from build123d import *

# Parameters (mm, degrees)
SKETCH1_R           = 2.1
SKETCH1_W           = 55.2
SKETCH1_H           = 5.05
BOSS_EXTRUDE1_DEPTH = 5
SKETCH2_W           = 55.4
SKETCH2_H           = 5.4
CUT_EXTRUDE1_DEPTH  = 10
SKETCH3_W           = 52.4
SKETCH3_H           = 5
CUT_EXTRUDE2_DEPTH  = 10
SKETCH4_W           = 40
SKETCH4_H           = 105
CUT_EXTRUDE3_DEPTH  = 10


with BuildPart() as part:
    # Sketch1 → Boss-Extrude1 (new body)
    with BuildSketch(Plane.XY):
        with BuildLine():
            Line((-192, 100.877501001), (-192, 60.122498999))
            ThreePointArc((-192, 60.122498999), (-193.5, 57), (-192, 53.877501001))
            Line((-192, 53.877501001), (-192, 13.122498999))
            ThreePointArc((-192, 13.122498999), (-193.5, 10), (-192, 6.877501001))
            Line((-192, 6.877501001), (-192, 0))
            Line((-192, 0), (-122, 0))
            Line((-122, 0), (-122, 5))
            Line((-122, 5), (-98.1, 5))
            Line((-98.1, 5), (-98.1, 11.8))
            Line((-98.1, 11.8), (-99.5, 11.8))
            Line((-99.5, 11.8), (-99.5, 15))
            Line((-99.5, 15), (-98.1, 15))
            Line((-98.1, 15), (-98.1, 22))
            Line((-98.1, 22), (-93.9, 22))
            Line((-93.9, 22), (-93.9, 15))
            Line((-93.9, 15), (-92.5, 15))
            Line((-92.5, 15), (-92.5, 11.8))
            Line((-92.5, 11.8), (-93.9, 11.8))
            Line((-93.9, 11.8), (-93.9, 5))
            Line((-93.9, 5), (-70, 5))
            Line((-70, 5), (-70, 0))
            Line((-70, 0), (0, 0))
            Line((0, 0), (0, 30.327501001))
            ThreePointArc((0, 30.327501001), (1.5, 33.45), (0, 36.572498999))
            Line((0, 36.572498999), (0, 77.327501001))
            ThreePointArc((0, 77.327501001), (1.5, 80.45), (0, 83.572498999))
            Line((0, 83.572498999), (0, 122.277501001))
            ThreePointArc((0, 122.277501001), (1.5, 125.4), (0, 128.522498999))
            Line((0, 128.522498999), (0, 160))
            Line((0, 160), (-32.9, 160))
            Line((-32.9, 160), (-32.9, 153.2))
            Line((-32.9, 153.2), (-31.5, 153.2))
            Line((-31.5, 153.2), (-31.5, 150))
            Line((-31.5, 150), (-32.9, 150))
            Line((-32.9, 150), (-32.9, 143))
            Line((-32.9, 143), (-37.1, 143))
            Line((-37.1, 143), (-37.1, 150))
            Line((-37.1, 150), (-38.5, 150))
            Line((-38.5, 150), (-38.5, 153.2))
            Line((-38.5, 153.2), (-37.1, 153.2))
            Line((-37.1, 153.2), (-37.1, 160))
            Line((-37.1, 160), (-154.9, 160))
            Line((-154.9, 160), (-154.9, 153.2))
            Line((-154.9, 153.2), (-153.5, 153.2))
            Line((-153.5, 153.2), (-153.5, 150))
            Line((-153.5, 150), (-154.9, 150))
            Line((-154.9, 150), (-154.9, 143))
            Line((-154.9, 143), (-159.1, 143))
            Line((-159.1, 143), (-159.1, 150))
            Line((-159.1, 150), (-160.5, 150))
            Line((-160.5, 150), (-160.5, 153.2))
            Line((-160.5, 153.2), (-159.1, 153.2))
            Line((-159.1, 153.2), (-159.1, 160))
            Line((-159.1, 160), (-192, 160))
            Line((-192, 160), (-192, 107.122498999))
            ThreePointArc((-192, 107.122498999), (-193.5, 104), (-192, 100.877501001))
        make_face()
        with Locations((-189.5, 104)):
            Circle(SKETCH1_R, mode=Mode.SUBTRACT)
        with Locations((-189.5, 57)):
            Circle(SKETCH1_R, mode=Mode.SUBTRACT)
        with Locations((-189.5, 10)):
            Circle(SKETCH1_R, mode=Mode.SUBTRACT)
        with Locations((-2.5, 125.4)):
            Circle(SKETCH1_R, mode=Mode.SUBTRACT)
        with Locations((-2.5, 80.45)):
            Circle(SKETCH1_R, mode=Mode.SUBTRACT)
        with Locations((-2.5, 33.45)):
            Circle(SKETCH1_R, mode=Mode.SUBTRACT)
        with Locations((-159.4, 127.475)):
            Rectangle(SKETCH1_W, SKETCH1_H, mode=Mode.SUBTRACT)
        with Locations((-159.4, 80.475)):
            Rectangle(SKETCH1_W, SKETCH1_H, mode=Mode.SUBTRACT)
        with Locations((-159.4, 33.475)):
            Rectangle(SKETCH1_W, SKETCH1_H, mode=Mode.SUBTRACT)
        with Locations((-32.6, 103.925)):
            Rectangle(SKETCH1_W, SKETCH1_H, mode=Mode.SUBTRACT)
        with Locations((-32.6, 56.925)):
            Rectangle(SKETCH1_W, SKETCH1_H, mode=Mode.SUBTRACT)
        with Locations((-32.6, 9.925)):
            Rectangle(SKETCH1_W, SKETCH1_H, mode=Mode.SUBTRACT)
    extrude(amount=BOSS_EXTRUDE1_DEPTH)

    # Sketch2 → Cut-Extrude1 (cut)
    with BuildSketch(Plane.XY.offset(5)):
        with Locations((-159.4, 127.475)):
            Rectangle(SKETCH2_W, SKETCH2_H)
        with Locations((-32.6, 103.925)):
            Rectangle(SKETCH2_W, SKETCH2_H)
        with Locations((-159.4, 80.525)):
            Rectangle(SKETCH2_W, SKETCH2_H)
        with Locations((-159.4, 37.347324844)):
            Rectangle(SKETCH2_W, SKETCH2_H)
        with Locations((-32.6, 56.975)):
            Rectangle(SKETCH2_W, SKETCH2_H)
        with Locations((-32.6, 9.925)):
            Rectangle(SKETCH2_W, SKETCH2_H)
    extrude(amount=-CUT_EXTRUDE1_DEPTH, mode=Mode.SUBTRACT)

    # Sketch3 → Cut-Extrude2 (cut)
    with BuildSketch(Plane.XY.offset(5)):
        with Locations((-96, 2.5)):
            Rectangle(SKETCH3_W, SKETCH3_H)
    extrude(amount=-CUT_EXTRUDE2_DEPTH, mode=Mode.SUBTRACT)

    # Sketch4 → Cut-Extrude3 (cut)
    with BuildSketch(Plane.XY.offset(5)):
        with Locations((-96, 82.5)):
            Rectangle(SKETCH4_W, SKETCH4_H)
    extrude(amount=-CUT_EXTRUDE3_DEPTH, mode=Mode.SUBTRACT)


solid = part.part
The model under review builds one solid part; all positions refer to its coordinate system, in mm. A direction names the side the tool comes from. Give positions to 0.01 mm unless a question says otherwise; leave off trailing zeros. Write each loop counter-clockwise with the first axis right and the second up, starting at its lowest first coordinate (ties: lowest second). Pieces come first, ordered by that corner, then holes. Notation, with made-up numbers: M 30.5,13 L 35.5,13 A22 cw 35.5,28 Z; hole C 14.25,52.5 d4. An arc over 180 degrees is marked long. One line per question, with ' | ' between items. Start each with the question number.
Item 1: For faces 4 (the flat face through (-192, 81, 2)), 5 (the flat face through (-98.1, 8, 2)), 6 (the flat face through (-4.9, 57, 3)), 7 (the flat face through (0, 57, 2)), list the 3-axis set-ups (+Z, -Z, +X, -X, +Y, -Y) from which the entire face can be reached by the end or side of a thin tool; tool diameter is ignored.
Item 2: Wall thickness on line 1 (Y direction, x = -2.5, z = 2.95); line 2 (Y direction, x = -189.5, z = 3.85); line 3 (Y direction, x = -110.5, z = 2.1): over which ranges is each line inside the solid? List them lowest first. Write a range as from..to.
Item 3: For pin 1 (3 mm diameter, centred on y = 140, z = 2, fed in from +X); pin 2 (1.5 mm diameter, centred on x = -87, z = 3.5, fed in from -Y); pin 3 (1.5 mm diameter, centred on y = 36.5, z = 3.5, fed in from -X); pin 4 (3.5 mm diameter, centred on x = -189.5, y = 104, fed in from -Z), all flat-tipped, find the tip position at first contact; note any pin that passes through.
Item 4: We need section D-D on z = 2.75. Give the number of separate pieces and of enclosed holes in the cut face, plus the area to 3 significant figures.
Item 5: We need section C-C on y = 19. Write out the cut boundary in (x, z).
Item 6: Draft analysis for pull direction Y (two halves, no side actions). For faces 1 (the flat face through (-35, 143, 2)), 2 (the flat face through (0, 15, 2)), 3 (the cylindrical face through (1.5, 33.4, 2.5)), state which applies: released by +Y, released by -Y, zero draft, split by the parting line, or undercut.
Item 7: We need section B-B on y = 57. Write out the cut boundary in (x, z), plus the area to 4 significant figures.
Item 8: We need section A-A on x = -11.5. Write out the cut boundary in (y, z) (3 decimals).
Results found:
1) face 4: +Z, -Z, -X | face 5: +Z, -Z, -Y | face 6: +Z, -Z | face 7: +Z, -Z, +X
2) line 1: y = 0..31.35, 35.55..78.35, 82.55..123.3, 127.5..160 | line 2: y = 0..7.9, 12.1..54.9, 59.1..101.9, 106.1..160 | line 3: y = 5..30, 135..160
3) pin 1: stops at x = 0 | pin 2: stops at y = 5 | pin 3: stops at x = -192 | pin 4: passes through
4) separate pieces: 1 | enclosed holes: 13 | area: 24,000 mm2
5) outline: M -192,0 L -98.1,0 L -98.1,5 L -192,5 Z; M -93.9,0 L 0,0 L 0,5 L -93.9,5 Z
6) face 1: released by +Y | face 2: zero draft | face 3: undercut
7) outline: M -193.5,0 L -191.6,0 L -191.6,5 L -193.5,5 Z; M -187.4,0 L -116,0 L -116,5 L -187.4,5 Z; M -76,0 L -60.3,0 L -60.3,5 L -76,5 Z; M -4.9,0 L 0,0 L 0,5 L -4.9,5 Z | area: 469.5 mm2
8) outline: M 0,0 L 7.225,0 L 7.225,5 L 0,5 Z; M 12.625,0 L 54.275,0 L 54.275,5 L 12.625,5 Z; M 59.675,0 L 101.225,0 L 101.225,5 L 59.675,5 Z; M 106.625,0 L 160,0 L 160,5 L 106.625,5 Z
